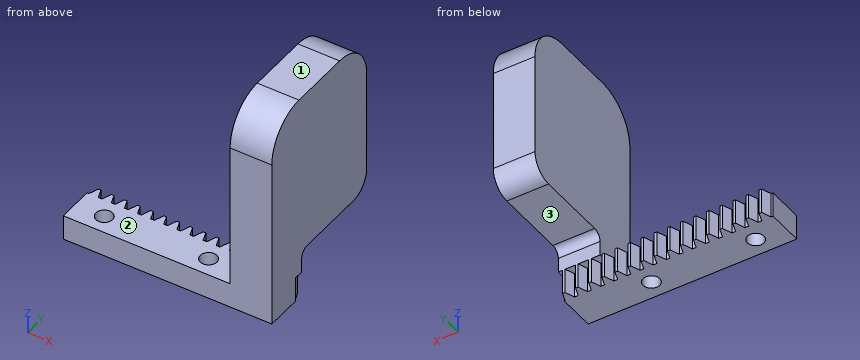
from build123d import *

# Parameters (mm, degrees)
BLANKSKE_W          = 50
BLANKSKE_H          = 11
BLANK_DEPTH         = 6
TOOTHCUTSIM_DEPTH   = 52.546095875
TEETHCUTS_COUNT     = 17
TEETHCUTS_PITCH     = 3.14159265
SKETCH1_W           = 10
SKETCH1_H           = 35
BOSS_EXTRUDE1_DEPTH = 45
FILLET1_R           = 10
SKETCH2_R           = 2
CUT_EXTRUDE1_DEPTH  = 25
SKETCH4_W           = 5.5
SKETCH4_H           = 30
CUT_EXTRUDE2_DEPTH  = 10
FILLET3_R           = 2
FILLET4_R           = 5


with BuildPart() as part:
    # BlankSke → Blank (new body)
    with BuildSketch(Plane.XY):
        with Locations((25, 5.5)):
            Rectangle(BLANKSKE_W, BLANKSKE_H)
    extrude(amount=-BLANK_DEPTH)

    # TooCutSkeSim → ToothCutSim (cut, through all)
    with BuildSketch(Plane.XY):
        Polygon((0.44443537, 8.75), (-0.44443537, 8.75), (-1.272613241, 11.0254), (1.272613241, 11.0254), align=None)
    toothcutsim = extrude(amount=-TOOTHCUTSIM_DEPTH, mode=Mode.SUBTRACT)

    # TeethCuts: ToothCutSim ×17
    with Locations(*[(i * TEETHCUTS_PITCH, 0, 0) for i in range(1, TEETHCUTS_COUNT)]):
        add(toothcutsim, mode=Mode.SUBTRACT)

    # Sketch1 → Boss-Extrude1 (add)
    with BuildSketch(Plane.XY):
        with Locations((45, 17.5)):
            Rectangle(SKETCH1_W, SKETCH1_H)
    extrude(amount=BOSS_EXTRUDE1_DEPTH)

    # Fillet1
    fillet1_edges = [part.edges().sort_by_distance(p)[0] for p in [
        (45, 35, 45),
        (45, 0, 45),
    ]]
    fillet(fillet1_edges, radius=FILLET1_R)

    # Sketch2 → Cut-Extrude1 (cut)
    with BuildSketch(Plane.XY):
        with Locations((7, 4.375)):
            Circle(SKETCH2_R)
        with Locations((32, 4.375)):
            Circle(SKETCH2_R)
    extrude(amount=-CUT_EXTRUDE1_DEPTH, mode=Mode.SUBTRACT)

    # Sketch4 → Cut-Extrude2 (cut)
    with BuildSketch(Plane.ZY.offset(-40)):
        with Locations((2.75, 26)):
            Rectangle(SKETCH4_W, SKETCH4_H)
    extrude(amount=-CUT_EXTRUDE2_DEPTH, mode=Mode.SUBTRACT)

    # Fillet3
    fillet3_edges = [part.edges().sort_by_distance(p)[0] for p in [
        (45, 11, 5.5),
    ]]
    fillet(fillet3_edges, radius=FILLET3_R)

    # Fillet4
    fillet4_edges = [part.edges().sort_by_distance(p)[0] for p in [
        (45, 35, 5.5),
    ]]
    fillet(fillet4_edges, radius=FILLET4_R)


solid = part.part
Here's how the part is built. I have some questions about the finished solid (model axes, mm). Face numbers are marked on the shaded views. A direction names the side the tool comes from. Coordinates: 2 decimals unless noted, no trailing zeros. Loops run counter-clockwise (first coordinate to the right, second up) from the corner with the lowest first, then second, coordinate; pieces in that order, holes last.
1. For the marked faces 1, 2 and 3, which set-ups out of +Z, -Z, +X, -X, +Y, -Y let a thin tool reach every point of the face, with its end or its side?
2. I need wall thicknesses on L1, parallel to X at y = 8, z = 6; L2, parallel to Y at x = 43, z = 35.5; L3, parallel to Z at x = 16, y = 2.5. Which ranges of each line are inside material? Lowest first, please.
3. Imagine slicing it at C-C, the plane z = -3. Count the separate pieces of the cut face and the enclosed holes in it, and give its area (3 significant figures).
4. Imagine slicing it at A-A, the plane z = 23.5. Please give me the cut outline in (x, y).
5. For P1, Ø0.5, axis at x = 23.5, z = -2, coming from the +Y side; P2, Ø10, axis at x = 5, y = 4.5, coming from the +Z side; P3, Ø10.5, axis at y = 15.5, z = 13.5, coming from the -X side, each with a flat end and sliding along its axis, tell me the tip position at first contact or that it passes through.
6. Imagine slicing it at B-B, the plane y = 21.5. Please give me the cut outline in (x, z), and give its area (3 significant figures).
Taken from the geometry:
1. face 1: +Z, +X, -X, +Y, -Y
1. face 2: +Z, -X, +Y, -Y
1. face 3: -Z, +X, -X, +Y
2. L1: x = 40 to 50
2. L2: y = 0.01 to 34.99
2. L3: z = -6 to 0
3. separate pieces: 1
3. enclosed holes: 2
3. area: 464 mm2
4. outline: (40, 0) - (50, 0) - (50, 35) - (40, 35) - close
5. P1: stops at y = 11
5. P2: stops at z = 0
5. P3: stops at x = 40
6. outline: (40, 5.5) - (50, 5.5) - (50, 45) - (40, 45) - close
6. area: 395 mm2
